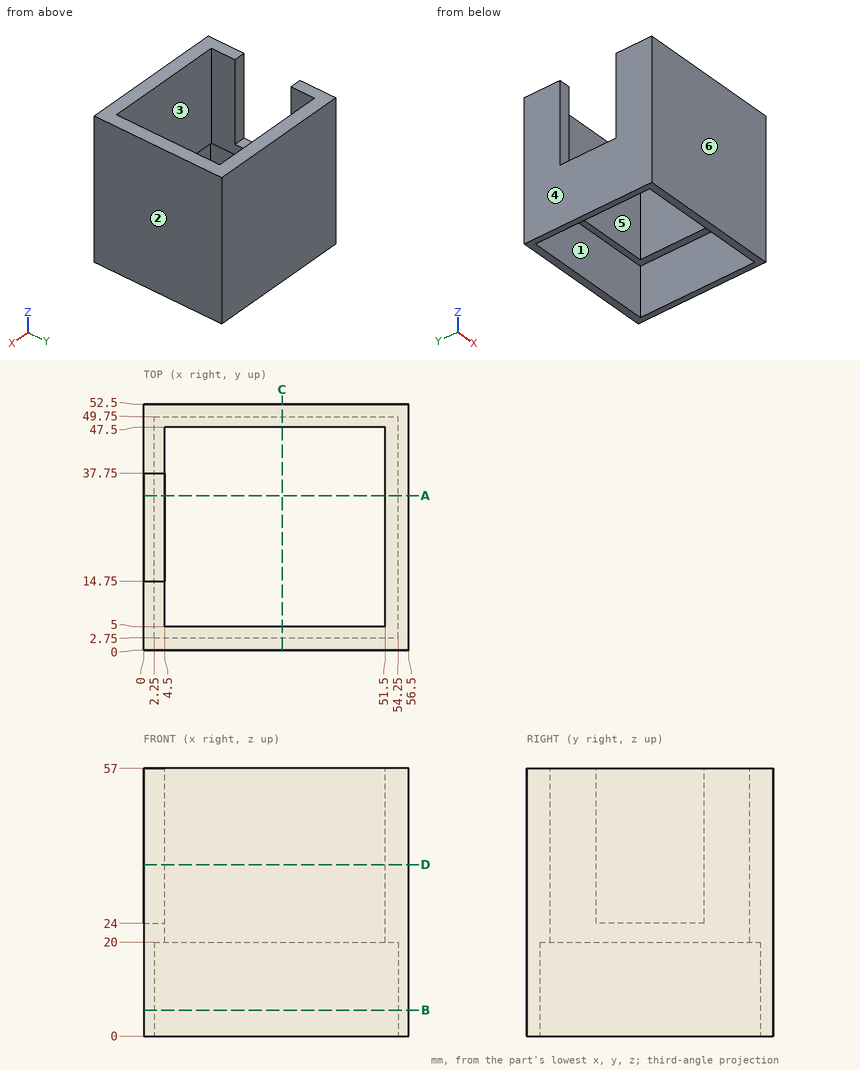
Study the drawing (mm; zero at the part's minimum x, y, z) and answer. A direction names the side the tool comes from. Give positions to 0.01 mm unless a question says otherwise; leave off trailing zeros. Loops run counter-clockwise (first coordinate to the right, second up) from the corner with the lowest first, then second, coordinate; pieces in that order, holes last. Notation, with made-up numbers: (76.5, -12.75) - (95.5, -12.75) arc R17 ccw to (95.5, 10.25) - close; hole circle Ø5 at (57.5, 87.5). An arc over 180 degrees is marked (long way). Use CSV: the item, a comma, the result in double quotes. Start each with the question number.
(1) Find the intervals of material crossed by L1, parallel to Y at x = 36, z = 18; L2, parallel to X at y = 46, z = 15.5; L3, parallel to X at y = 40, z = 40, in increasing order.
(2) Determine the mould class of the marked faces 4, 5 and 6 for opening direction X: released by +X, released by -X, zero draft, split by the parting line, or undercut.
(3) Each of these flat-tipped pins is pushed along its axis until it touches: pin 1 (1.5 mm diameter, centred on y = 24.5, z = 40.5, fed in from -X); pin 2 (5 mm diameter, centred on x = 1.5, y = 22, fed in from +Z). Where does it stop, or does it pass through?
(4) A tool of negligible diameter and unlimited length cuts with its end or side. For the marked faces 1, 2 and 3, from which of +Z, -Z, +X, -X, +Y, -Y can it reach the whole face along a straight path? Write none if from no direction.
(5) Find section B-B, the plane z = 5.5. Determine the outline of the cut face in (x, y).
(6) Find section A-A, the plane y = 33. Determine the outline of the cut face in (x, z), plus the area to 3 significant figures.
(7) Find section D-D, the plane z = 36.5. Determine the outline of the cut face in (x, y), plus the area to 3 significant figures.
(8) Find section C-C, the plane x = 29.5. Determine the outline of the cut face in (y, z).
Results found:
1,L1,"0 to 2.75, 49.75 to 52.5"
1,L2,"0 to 2.25, 54.25 to 56.5"
1,L3,"0 to 4.5, 51.5 to 56.5"
2,face 4,"released by -X"
2,face 5,"undercut"
2,face 6,"zero draft"
3,pin 1,"x = 51.5"
3,pin 2,"z = 24"
4,face 1,"-Z"
4,face 2,"+Z, -Z, +X, +Y, -Y"
4,face 3,"+Z, -Z"
5,outline,"(0, 0) - (56.5, 0) - (56.5, 52.5) - (0, 52.5) - close; hole (2.25, 2.75) - (54.25, 2.75) - (54.25, 49.75) - (2.25, 49.75) - close"
6,outline,"(0, 0) - (2.25, 0) - (2.25, 20) - (4.5, 20) - (4.5, 24) - (0, 24) - close; (51.5, 20) - (54.25, 20) - (54.25, 0) - (56.5, 0) - (56.5, 57) - (51.5, 57) - close"
6,area,"293 mm^2"
7,outline,"(0, 0) - (56.5, 0) - (56.5, 52.5) - (0, 52.5) - (0, 37.75) - (4.5, 37.75) - (4.5, 47.5) - (51.5, 47.5) - (51.5, 5) - (4.5, 5) - (4.5, 14.75) - (0, 14.75) - close"
7,area,"865 mm^2"
8,outline,"(0, 0) - (2.75, 0) - (2.75, 20) - (5, 20) - (5, 57) - (0, 57) - close; (47.5, 20) - (49.75, 20) - (49.75, 0) - (52.5, 0) - (52.5, 57) - (47.5, 57) - close"
